from build123d import *

# Parameters (mm, degrees)
SKETCH1_W           = 30
SKETCH1_H           = 72.5
BOSS_EXTRUDE1_DEPTH = 15
SKETCH2_W           = 20.5
SKETCH2_H           = 41
CUT_EXTRUDE1_DEPTH  = 8
SKETCH3_W           = 30
SKETCH3_H           = 35
CUT_EXTRUDE2_DEPTH  = 9
CUT_EXTRUDE3_DEPTH  = 50.386865663
CUT_EXTRUDE4_REACH  = 44.001
SKETCH5_R           = 1.6
SKETCH6_R           = 3
CUT_EXTRUDE5_DEPTH  = 50.386865663
CUT_EXTRUDE6_REACH  = 44.001
SKETCH7_R           = 1.6
SKETCH8_W           = 7
SKETCH8_H           = 7
BOSS_EXTRUDE2_DEPTH = 4.5
CUT_EXTRUDE7_REACH  = 79.235
SKETCH9_R           = 1.6


with BuildPart() as part:
    # Sketch1 → Boss-Extrude1 (new body)
    with BuildSketch(Plane(origin=(0, 0, 0), x_dir=(1, 0, 0), z_dir=(0, 1, 0))):
        Rectangle(SKETCH1_W, SKETCH1_H)
    extrude(amount=BOSS_EXTRUDE1_DEPTH)

    # Sketch2 → Cut-Extrude1 (cut)
    with BuildSketch(Plane.XZ):
        with Locations((-0.25, 9)):
            Rectangle(SKETCH2_W, SKETCH2_H)
    extrude(amount=-CUT_EXTRUDE1_DEPTH, mode=Mode.SUBTRACT)

    # Sketch3 → Cut-Extrude2 (cut)
    with BuildSketch(Plane(origin=(0, 15, 0), x_dir=(1, 0, 0), z_dir=(0, 1, 0))):
        with Locations((0, 1.25)):
            Rectangle(SKETCH3_W, SKETCH3_H)
    extrude(amount=-CUT_EXTRUDE2_DEPTH, mode=Mode.SUBTRACT)

    # Sketch4 → Cut-Extrude3 (cut, through all)
    with BuildSketch(Plane(origin=(15, 0, 0), x_dir=(0, 0, -1), z_dir=(1, 0, 0))):
        Polygon((-33.75, 15), (-33.75, 10), (-27.25, 10), (-27.25, 5), (-36.25, 5), (-36.25, 15), align=None)
    extrude(amount=-CUT_EXTRUDE3_DEPTH, mode=Mode.SUBTRACT)

    # Sketch5 → Cut-Extrude4 (cut, up to next)
    with BuildSketch(Plane.XZ, mode=Mode.PRIVATE) as cut_extrude4_sk1:
        with Locations(Location((-5, 33, 0), (0, 0, 270))):
            Circle(SKETCH5_R)
    cut_extrude4_tool1 = extrude(cut_extrude4_sk1.sketch, amount=-CUT_EXTRUDE4_REACH, mode=Mode.PRIVATE) & part.part
    # Sketch5 → Cut-Extrude4 (cut, up to next)
    with BuildSketch(Plane.XZ, mode=Mode.PRIVATE) as cut_extrude4_sk2:
        with Locations(Location((5, 33, 0), (0, 0, 270))):
            Circle(SKETCH5_R)
    cut_extrude4_tool2 = extrude(cut_extrude4_sk2.sketch, amount=-CUT_EXTRUDE4_REACH, mode=Mode.PRIVATE) & part.part
    # Sketch5 → Cut-Extrude4 (cut, up to next)
    with BuildSketch(Plane.XZ, mode=Mode.PRIVATE) as cut_extrude4_sk3:
        with Locations(Location((-5, -15, 0), (0, 0, 270))):
            Circle(SKETCH5_R)
    cut_extrude4_tool3 = extrude(cut_extrude4_sk3.sketch, amount=-CUT_EXTRUDE4_REACH, mode=Mode.PRIVATE) & part.part
    # Sketch5 → Cut-Extrude4 (cut, up to next)
    with BuildSketch(Plane.XZ, mode=Mode.PRIVATE) as cut_extrude4_sk4:
        with Locations(Location((5, -15, 0), (0, 0, 270))):
            Circle(SKETCH5_R)
    cut_extrude4_tool4 = extrude(cut_extrude4_sk4.sketch, amount=-CUT_EXTRUDE4_REACH, mode=Mode.PRIVATE) & part.part
    add(cut_extrude4_tool1.solids().sort_by_distance((-5, 0, 33))[0], mode=Mode.SUBTRACT)
    add(cut_extrude4_tool2.solids().sort_by_distance((5, 0, 33))[0], mode=Mode.SUBTRACT)
    add(cut_extrude4_tool3.solids().sort_by_distance((-5, 0, -15))[0], mode=Mode.SUBTRACT)
    add(cut_extrude4_tool4.solids().sort_by_distance((5, 0, -15))[0], mode=Mode.SUBTRACT)

    # Sketch6 → Cut-Extrude5 (cut, through all)
    with BuildSketch(Plane(origin=(15, 0, 0), x_dir=(0, 0, -1), z_dir=(1, 0, 0))):
        with Locations((24.25, 14)):
            Circle(SKETCH6_R)
        with Locations((-21.75, 14)):
            Circle(SKETCH6_R)
    extrude(amount=-CUT_EXTRUDE5_DEPTH, mode=Mode.SUBTRACT)

    # Sketch7 → Cut-Extrude6 (cut, up to next)
    with BuildSketch(Plane(origin=(0, 15, 0), x_dir=(1, 0, 0), z_dir=(0, 1, 0)), mode=Mode.PRIVATE) as cut_extrude6_sk1:
        with Locations(Location((-9.5, -30.25, 0), (0, 0, 270))):
            Circle(SKETCH7_R)
    cut_extrude6_tool1 = extrude(cut_extrude6_sk1.sketch, amount=-CUT_EXTRUDE6_REACH, mode=Mode.PRIVATE) & part.part
    # Sketch7 → Cut-Extrude6 (cut, up to next)
    with BuildSketch(Plane(origin=(0, 15, 0), x_dir=(1, 0, 0), z_dir=(0, 1, 0)), mode=Mode.PRIVATE) as cut_extrude6_sk2:
        with Locations(Location((9.5, -30.25, 0), (0, 0, 270))):
            Circle(SKETCH7_R)
    cut_extrude6_tool2 = extrude(cut_extrude6_sk2.sketch, amount=-CUT_EXTRUDE6_REACH, mode=Mode.PRIVATE) & part.part
    # Sketch7 → Cut-Extrude6 (cut, up to next)
    with BuildSketch(Plane(origin=(0, 15, 0), x_dir=(1, 0, 0), z_dir=(0, 1, 0)), mode=Mode.PRIVATE) as cut_extrude6_sk3:
        with Locations(Location((-9.5, 31.55, 0), (0, 0, 270))):
            Circle(SKETCH7_R)
    cut_extrude6_tool3 = extrude(cut_extrude6_sk3.sketch, amount=-CUT_EXTRUDE6_REACH, mode=Mode.PRIVATE) & part.part
    # Sketch7 → Cut-Extrude6 (cut, up to next)
    with BuildSketch(Plane(origin=(0, 15, 0), x_dir=(1, 0, 0), z_dir=(0, 1, 0)), mode=Mode.PRIVATE) as cut_extrude6_sk4:
        with Locations(Location((9.5, 31.55, 0), (0, 0, 270))):
            Circle(SKETCH7_R)
    cut_extrude6_tool4 = extrude(cut_extrude6_sk4.sketch, amount=-CUT_EXTRUDE6_REACH, mode=Mode.PRIVATE) & part.part
    add(cut_extrude6_tool1.solids().sort_by_distance((-9.5, 15, 30.25))[0], mode=Mode.SUBTRACT)
    add(cut_extrude6_tool2.solids().sort_by_distance((9.5, 15, 30.25))[0], mode=Mode.SUBTRACT)
    add(cut_extrude6_tool3.solids().sort_by_distance((-9.5, 15, -31.55))[0], mode=Mode.SUBTRACT)
    add(cut_extrude6_tool4.solids().sort_by_distance((9.5, 15, -31.55))[0], mode=Mode.SUBTRACT)

    # Sketch8 → Boss-Extrude2 (add)
    with BuildSketch(Plane(origin=(0, 0, -36.25), x_dir=(-1, 0, 0), z_dir=(0, 0, -1))):
        with Locations((18.5, 11.5)):
            Rectangle(SKETCH8_W, SKETCH8_H)
        with Locations((-18.5, 11.5)):
            Rectangle(SKETCH8_W, SKETCH8_H)
    extrude(amount=-BOSS_EXTRUDE2_DEPTH)

    # Sketch9 → Cut-Extrude7 (cut, up to next)
    with BuildSketch(Plane(origin=(0, 0, -36.25), x_dir=(-1, 0, 0), z_dir=(0, 0, -1)), mode=Mode.PRIVATE) as cut_extrude7_sk1:
        with Locations((18.5, 11.5)):
            Circle(SKETCH9_R)
    cut_extrude7_tool1 = extrude(cut_extrude7_sk1.sketch, amount=-CUT_EXTRUDE7_REACH, mode=Mode.PRIVATE) & part.part
    # Sketch9 → Cut-Extrude7 (cut, up to next)
    with BuildSketch(Plane(origin=(0, 0, -36.25), x_dir=(-1, 0, 0), z_dir=(0, 0, -1)), mode=Mode.PRIVATE) as cut_extrude7_sk2:
        with Locations((-18.5, 11.5)):
            Circle(SKETCH9_R)
    cut_extrude7_tool2 = extrude(cut_extrude7_sk2.sketch, amount=-CUT_EXTRUDE7_REACH, mode=Mode.PRIVATE) & part.part
    add(cut_extrude7_tool1.solids().sort_by_distance((-18.5, 11.5, -36.25))[0], mode=Mode.SUBTRACT)
    add(cut_extrude7_tool2.solids().sort_by_distance((18.5, 11.5, -36.25))[0], mode=Mode.SUBTRACT)


solid = part.part
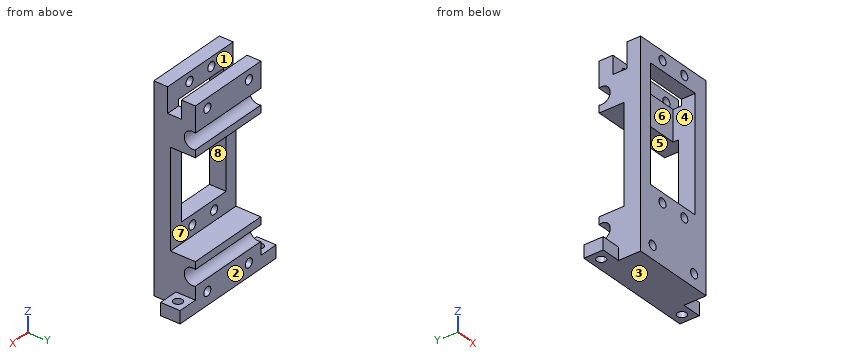
Source: CAD feature listing. Evaluate the final solid. Frame: model axes, mm. Face numbers are marked on the shaded views. A direction names the side the tool comes from. Give positions to 0.01 mm unless a question says otherwise; leave off trailing zeros. Order: outer loops, then holes, each group sorted by start corner. A loop starts at its lowest first (then second) coordinate and runs counter-clockwise, first axis right, second up. Notation, with made-up numbers: (38, -9.5) -> (59, -9.5) arc R32 cw to (59, 22.5) -> close; hole circle Ø8 at (-6.75, -39.75). An arc over 180 degrees is marked (long way). Write item = value, one per line.
Q1. Cut plane C-C, the plane y = 4.25. Output: boundary loops of the cut face in (x, z), and give its area (3 significant figures).
Data:
outline = (-15, -36.25) -> (15, -36.25) -> (15, 36.25) -> (-15, 36.25) -> close; hole circle Ø3.2 at (-9.5, -31.55); hole (-10.5, -11.5) -> (10, -11.5) -> (10, 29.5) -> (-10.5, 29.5) -> close; hole circle Ø3.2 at (-5, -15); hole circle Ø3.2 at (-5, 33); hole circle Ø3.2 at (5, -15); hole circle Ø3.2 at (5, 33); hole circle Ø3.2 at (9.5, -31.55)
area = 1,290 mm^2
Q2. Cut plane D-D, the plane x = 1.5. Output: boundary loops of the cut face in (y, z).
Data:
outline = (0, -36.25) -> (15, -36.25) -> (15, -27.08) arc R3 cw (long way) to (15, -21.42) -> (15, -18.75) -> (6, -18.75) -> (6, -11.5) -> (0, -11.5) -> close; (0, 29.5) -> (5, 29.5) -> (5, 36.25) -> (0, 36.25) -> close; (8, 16.25) -> (15, 16.25) -> (15, 18.92) arc R3 cw (long way) to (15, 24.58) -> (15, 33.75) -> (10, 33.75) -> (10, 27.25) -> (8, 27.25) -> close
Q3. Pin query (flat end, axial travel): pin 1 (1.9 mm diameter, centred on x = -9.5, z = 30.25, fed in from +Y); pin 2 (4 mm diameter, centred on x = -6.5, y = 13, fed in from +Z); pin 3 (5 mm diameter, centred on y = 6, z = 22.5, fed in from +X); pin 4 (2 mm diameter, centred on x = -17.5, y = 2, fed in from +Z). Return the tip coordinate at first contact, or that it passes through.
Data:
pin_1 = 5
pin_2 = 33.75
pin_3 = 15
pin_4 = through
Q4. Set-up query: the marked faces 1, 2, 3, 4 and 5. Return all of +Z, -Z, +X, -X, +Y, -Y with unobstructed straight access to the full face (end or side cutting, diameter ignored); none if empty.
Data:
face_1 = +Z, +X, -X
face_2 = +Z, -Z, +X, -X, +Y
face_3 = -Z, +X, -X, +Y, -Y
face_4 = -Y
face_5 = +X, -X, +Y
Q5. Material intervals for line 1 (X direction, y = 3.4, z = -15); line 2 (Z direction, x = 6, y = 14); line 3 (X direction, y = 5.5, z = -9), sorted ascending. Write a range as from..to.
Data:
line_1 = -15..-6.6, -3.4..3.4, 6.6..15
line_2 = -36.25..-27.25, -21.25..-18.75, 16.25..18.75, 24.75..33.75
line_3 = -15..-10.5, 10..15
Q6. Cut plane B-B, the plane x = -9.5. Output: boundary loops of the cut face in (y, z).
Data:
outline = (0, -36.25) -> (15, -36.25) -> (15, -33.15) -> (0, -33.15) -> close; (0, -29.95) -> (15, -29.95) -> (15, -27.08) arc R3 cw (long way) to (15, -21.42) -> (15, -18.75) -> (6, -18.75) -> (6, -11.5) -> (0, -11.5) -> close; (0, 29.5) -> (5, 29.5) -> (5, 36.25) -> (0, 36.25) -> close; (8, 16.25) -> (15, 16.25) -> (15, 18.92) arc R3 cw (long way) to (15, 24.58) -> (15, 28.65) -> (10, 28.65) -> (10, 27.25) -> (8, 27.25) -> close; (10, 31.85) -> (15, 31.85) -> (15, 33.75) -> (10, 33.75) -> close
Q7. Pull-direction query (X, two-part tool) for the marked faces 6, 7 and 8; classes: released by +X, released by -X, zero draft, split by the parting line, or undercut.
Data:
face_6 = undercut
face_7 = zero draft
face_8 = undercut
Q8. Cut plane A-A, the plane z = 8. Output: boundary loops of the cut face in (x, y), and give its area (3 significant figures).
Data:
outline = (-15, 0) -> (-10.5, 0) -> (-10.5, 6) -> (-15, 6) -> close; (10, 0) -> (15, 0) -> (15, 6) -> (10, 6) -> close
area = 57.0 mm^2
